```python
from build123d import *

# Parameters (mm, degrees)
SZKIC1_W                     = 60
SZKIC1_H                     = 60
DODANIE_WYCI_GNI_CIE1_DEPTH  = 80
SZKIC2_W                     = 57.5
SZKIC2_H                     = 57.5
WYTNIJ_WYCI_GNI_CIE1_DEPTH   = 6
SZKIC3_R                     = 5
WYTNIJ_WYCI_GNI_CIE2_DEPTH   = 24
SZKIC4_R                     = 19
WYTNIJ_WYCI_GNI_CIE3_DEPTH   = 0.9
ZAOKR_GLENIE1_R              = 1
OTWORY_USTALAJ_CE_6_0MM1_D   = 6
SZKIC8_R                     = 21
WYTNIJ_WYCI_GNI_CIE5_DEPTH   = 70
ZAOKR_GLENIE2_R              = 1
OTW_R_POD_RUB_M81_AT_2_COUNT = 2
OTW_R_POD_RUB_M81_AT_2_PITCH = 30
OTW_R_POD_RUB_M81_AT_3_COUNT = 2
OTW_R_POD_RUB_M81_AT_3_PITCH = 50
OTW_R_POD_RUB_M81_AT_4_COUNT = 2
OTW_R_POD_RUB_M81_AT_4_PITCH = 40


with BuildPart() as part:
    # Szkic1 → Dodanie-wyciągnięcie1 (new body)
    with BuildSketch(Plane(origin=(0, 0, 0), x_dir=(1, 0, 0), z_dir=(0, 1, 0))):
        Rectangle(SZKIC1_W, SZKIC1_H)
    extrude(amount=DODANIE_WYCI_GNI_CIE1_DEPTH)

    # Szkic2 → Wytnij-wyciągnięcie1 (cut)
    with BuildSketch(Plane(origin=(0, 80, 0), x_dir=(1, 0, 0), z_dir=(0, 1, 0))):
        Rectangle(SZKIC2_W, SZKIC2_H)
    extrude(amount=-WYTNIJ_WYCI_GNI_CIE1_DEPTH, mode=Mode.SUBTRACT)

    # Szkic3 → Wytnij-wyciągnięcie2 (cut)
    with BuildSketch(Plane(origin=(0, 74, 0), x_dir=(1, 0, 0), z_dir=(0, 1, 0))):
        with Locations(Location((0, 0, 0), (0, 0, 270))):
            Circle(SZKIC3_R)
    extrude(amount=-WYTNIJ_WYCI_GNI_CIE2_DEPTH, mode=Mode.SUBTRACT)

    # Szkic4 → Wytnij-wyciągnięcie3 (cut)
    with BuildSketch(Plane(origin=(0, 74, 0), x_dir=(1, 0, 0), z_dir=(0, 1, 0))):
        with Locations(Location((0, 0, 0), (0, 0, 270))):
            Circle(SZKIC4_R)
    extrude(amount=-WYTNIJ_WYCI_GNI_CIE3_DEPTH, mode=Mode.SUBTRACT)

    # Zaokrąglenie1
    # the kernel refuses this fillet: 1 mm, written as the material it adds along each edge
    with BuildSketch(Plane(origin=(0, 73.1, 0), x_dir=(0, 0, 1), z_dir=(-1, 0, 0))) as zaokr_glenie1_piece_1:
        with BuildLine():
            CenterArc((18.005012563, 1), ZAOKR_GLENIE1_R, 270, 84.260829523)
            Line((18.005012563, 0), (18.005012563, -0.02))
            Line((18.005012563, -0.02), (19, -0.02))
            Line((19, -0.02), (19.02, 0))
            ThreePointArc((19.02, 0), (19.02, 0.45), (19.019899749, 0.898))
            Line((19.019899749, 0.898), (19, 0.9))
        make_face()
    revolve(axis=Axis((0, 73.1, 0), (0, 1, 0)))

    # Otwory ustalające Ø6.0mm1 (through all)
    with Locations(Plane(origin=(0, 74, 0), x_dir=(1, 0, 0), z_dir=(0, 1, 0))):
        with Locations((-24, 24), (24, 24), (24, -24), (-24, -24)):
            Hole(OTWORY_USTALAJ_CE_6_0MM1_D / 2)

    # Szkic8 → Wytnij-wyciągnięcie5 (cut)
    with BuildSketch(Plane.XZ):
        with Locations(Location((0, 0, 0), (0, 0, 270))):
            Circle(SZKIC8_R)
    extrude(amount=-WYTNIJ_WYCI_GNI_CIE5_DEPTH, mode=Mode.SUBTRACT)

    # Zaokrąglenie2
    zaokr_glenie2_edges = [part.edges().sort_by_distance(p)[0] for p in [
        (30, 80, 0),
        (0, 80, -30),
        (-30, 80, 0),
        (0, 0, -30),
        (30, 0, 0),
        (0, 0, 30),
        (-30, 0, 0),
        (-30, 40, -30),
        (30, 40, -30),
        (30, 40, 30),
        (-30, 40, 30),
        (0, 80, 30),
    ]]
    fillet(zaokr_glenie2_edges, radius=ZAOKR_GLENIE2_R)

    # Szkic11 → Otwór pod śrubę M81 (revolve, cut)
    with BuildSketch(Plane(origin=(15, 60, -30), x_dir=(0, 1, 0), z_dir=(1, 0, 0))):
        Polygon((0, 0), (0, 12.703872786), (4.5, 10), (4.5, 0), align=None)
    otw_r_pod_rub_m81 = revolve(axis=Axis((15, 60, -36.35), (0, 0, 1)), mode=Mode.SUBTRACT)

    # Otwór pod śrubę M81 at 2: Otwór pod śrubę M81 ×2
    with Locations(*[(-i * OTW_R_POD_RUB_M81_AT_2_PITCH, 0, 0) for i in range(1, OTW_R_POD_RUB_M81_AT_2_COUNT)]):
        add(otw_r_pod_rub_m81, mode=Mode.SUBTRACT)

    # Otwór pod śrubę M81 at 3: Otwór pod śrubę M81 ×2
    with Locations(*[Vector(-0.6, -0.8000000000000002, 0) * (i * OTW_R_POD_RUB_M81_AT_3_PITCH) for i in range(1, OTW_R_POD_RUB_M81_AT_3_COUNT)]):
        add(otw_r_pod_rub_m81, mode=Mode.SUBTRACT)

    # Otwór pod śrubę M81 at 4: Otwór pod śrubę M81 ×2
    with Locations(*[(0, -i * OTW_R_POD_RUB_M81_AT_4_PITCH, 0) for i in range(1, OTW_R_POD_RUB_M81_AT_4_COUNT)]):
        add(otw_r_pod_rub_m81, mode=Mode.SUBTRACT)

    # Lustro1: Otwór pod śrubę M81 across plane
    add(otw_r_pod_rub_m81.mirror(Plane.XY), mode=Mode.SUBTRACT)

    # Lustro1 copy 1 sketch → Lustro1 copy 1 (revolve, cut)
    with BuildSketch(Plane(origin=(-15, 60, 30), x_dir=(0, 1, 0), z_dir=(1, 0, 0))):
        Polygon((0, 0), (0, -12.703872786), (4.5, -10), (4.5, 0), align=None)
    revolve(axis=Axis((-15, 60, 36.35), (0, 0, 1)), mode=Mode.SUBTRACT)

    # Lustro1 copy 2 sketch → Lustro1 copy 2 (revolve, cut)
    with BuildSketch(Plane(origin=(-15, 20, 30), x_dir=(0, 1, 0), z_dir=(1, 0, 0))):
        Polygon((0, 0), (0, -12.703872786), (4.5, -10), (4.5, 0), align=None)
    revolve(axis=Axis((-15, 20, 36.35), (0, 0, 1)), mode=Mode.SUBTRACT)

    # Lustro1 copy 3 sketch → Lustro1 copy 3 (revolve, cut)
    with BuildSketch(Plane(origin=(15, 20, 30), x_dir=(0, 1, 0), z_dir=(1, 0, 0))):
        Polygon((0, 0), (0, -12.703872786), (4.5, -10), (4.5, 0), align=None)
    revolve(axis=Axis((15, 20, 36.35), (0, 0, 1)), mode=Mode.SUBTRACT)


solid = part.part
```
Source: CAD feature listing. Evaluate the final solid. Frame: model axes, mm. A direction names the side the tool comes from. Round coordinates to 2 decimals unless told otherwise and drop trailing zeros. Loops run counter-clockwise (first coordinate to the right, second up) from the corner with the lowest first, then second, coordinate; pieces in that order, holes last. Notation, with made-up numbers: (-22.5, 80.25) - (22.5, 80.25) arc R34 ccw to (22.5, 114.25) - close; hole circle Ø2 at (26.5, -22.75). An arc over 180 degrees is marked (long way). Use CSV: the item, a comma, the result in double quotes.
Q1. Section query D-D, the plane z = 0. Output: boundary loops of the cut face in (x, y).
Reported:
outline,"(-30, 1) arc R1 ccw to (-29, 0) - (-21, 0) - (-21, 70) - (-5, 70) - (-5, 73.1) - (-18.01, 73.1) arc R1 cw to (-19, 74) - (-28.75, 74) - (-28.75, 80) - (-29, 80) arc R1 ccw to (-30, 79) - close; (5, 70) - (21, 70) - (21, 0) - (29, 0) arc R1 ccw to (30, 1) - (30, 79) arc R1 ccw to (29, 80) - (28.75, 80) - (28.75, 74) - (19, 74) arc R1 cw to (18.01, 73.1) - (5, 73.1) - close"
Q2. Ray query, line 1 along Y through (x, z) = (15, -24.5); line 2 along X through (y, z) = (60, 24); line 3 along X through (y, z) = (42, -24). Return the intervals inside material, ascending.
Reported:
line 1,"0 to 15.5, 24.5 to 55.5, 64.5 to 74"
line 2,"-30 to -27, -21 to -19.5, -10.5 to 10.5, 19.5 to 21, 27 to 30"
line 3,"-30 to -27, -21 to 21, 27 to 30"
Q3. Section query B-B, the plane y = 75.5. Output: boundary loops of the cut face in (x, z).
Reported:
outline,"(-30, -29) arc R1 ccw to (-29, -30) - (29, -30) arc R1 ccw to (30, -29) - (30, 29) arc R1 ccw to (29, 30) - (-29, 30) arc R1 ccw to (-30, 29) - close; hole (-28.75, -28.75) - (28.75, -28.75) - (28.75, 28.75) - (-28.75, 28.75) - close"
Q4. Section query A-A, the plane z = -24. Output: boundary loops of the cut face in (x, y), then the cut area to 3 significant figures.
Reported:
outline,"(-30, 1) arc R1 ccw to (-29, 0) - (-27, 0) - (-27, 74) - (-28.75, 74) - (-28.75, 80) - (-29, 80) arc R1 ccw to (-30, 79) - close; (-21, 0) - (21, 0) - (21, 74) - (-21, 74) - close; (27, 0) - (29, 0) arc R1 ccw to (30, 1) - (30, 79) arc R1 ccw to (29, 80) - (28.75, 80) - (28.75, 74) - (27, 74) - close; hole circle Ø9 at (-15, 20); hole circle Ø9 at (-15, 60); hole circle Ø9 at (15, 20); hole circle Ø9 at (15, 60)"
area,"3,310 mm^2"
Q5. Mould query, pull axis X, two halves, no side actions, for faces 1 (the flat face through (-13, 0, -20)), 2 (the conical face through (-15.53, 59.42, -17.77)), 3 (the flat face through (-30, 39, 0)). Classes: pulls with the +X half, pulls with the -X half, needs draft (parallel to the pull), parting line crosses it, or undercut.
Reported:
face 1,"needs draft"
face 2,"undercut"
face 3,"pulls with the -X half"
Q6. Section query C-C, the plane x = 24. Output: boundary loops of the cut face in (y, z), then the cut area to 3 significant figures.
Reported:
outline,"(0, -29) arc R1 ccw to (1, -30) - (79, -30) arc R1 ccw to (80, -29) - (80, -28.75) - (74, -28.75) - (74, -27) - (0, -27) - close; (0, -21) - (74, -21) - (74, 21) - (0, 21) - close; (0, 27) - (74, 27) - (74, 28.75) - (80, 28.75) - (80, 29) arc R1 ccw to (79, 30) - (1, 30) arc R1 ccw to (0, 29) - close"
area,"3,570 mm^2"
Q7. Reachability of faces 4 (the flat face through (0, 39, -30)), 5 (the cylindrical face through (-18.794, 62.419, -25.07)), 6 (the flat face through (0, 77, -28.75)), 7 (the cylindrical face through (6.31, 34.51, -20.03)), 8 (the cylindrical face through (-18.04, 16.68, 25.07)) from +Z, -Z, +X, -X, +Y, -Y: full face, straight path, thin tool, end or side. Return the list, or none.
Reported:
face 4,"-Z, +X, -X, +Y, -Y"
face 5,"-Z"
face 6,"+Y"
face 7,"-Y"
face 8,"+Z"
Q8. Pin query (flat end, axial travel): pin 1 Ø21 at (x, z) = (-6.5, -1.5) entering from -Y; pin 2 Ø3 at (x, z) = (-13, 20.5) entering from +Y; pin 3 Ø5.5 at (x, z) = (24, -24) entering from -Y; pin 4 Ø7 at (x, y) = (15, 20) entering from +Z. Return the tip coordinate at first contact, or that it passes through.
Reported:
pin 1,"y = 70"
pin 2,"y = 74"
pin 3,"through"
pin 4,"z = 19.4"
